The listing builds one solid part. Answer for the finished solid, in the listing's coordinates (mm). Coordinates: 2 decimals unless noted, no trailing zeros. Loops run counter-clockwise (first coordinate to the right, second up) from the corner with the lowest first, then second, coordinate; pieces in that order, holes last. Notation, with made-up numbers: (-2.75, -14.5) - (52.25, -14.5) arc R23 ccw to (52.25, 24.5) - close; hole circle Ø9 at (-29, 34.25). An arc over 180 degrees is marked (long way). Use one line per item in the form item = value. Start each with the question number.
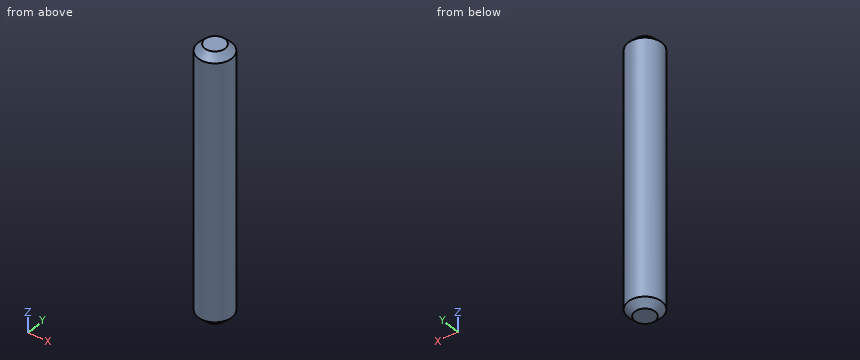
```python
from build123d import *

# Parameters (mm, degrees)
SKETCH_1_R      = 2.5
EXTRUDE_1_DEPTH = 40
CHAMFER_1_SIZE  = 1
CHAMFER_2_SIZE  = 1


with BuildPart() as part:
    # Эскиз1 → Бобышка-Вытянуть1 (new body)
    with BuildSketch(Plane.XY):
        Circle(SKETCH_1_R)
    extrude(amount=EXTRUDE_1_DEPTH)

    # Фаска1
    chamfer_1_edges = [part.edges().sort_by_distance(p)[0] for p in [
        (-2.5, 0, 40),
    ]]
    chamfer(chamfer_1_edges, length=CHAMFER_1_SIZE)

    # Фаска2
    chamfer_2_edges = [part.edges().sort_by_distance(p)[0] for p in [
        (-2.5, 0, 0),
    ]]
    chamfer(chamfer_2_edges, length=CHAMFER_2_SIZE)


solid = part.part
```
(1) Find the intervals of material crossed by probe 1 along X at (y, z) = (0.2, 27); probe 2 along Z at (x, y) = (-1.15, -2); probe 3 along Z at (x, y) = (-1.9, 0.8), in increasing order. Write a range as from..to.
(2) This flat-tipped pin is pushed along its axis until it touches: pin 1 Ø3 at (x, y) = (2, -1) entering from -Z. Where does it stop, or does it pass through?
(3) A cutting plane is placed at A-A (z = 3). Determine the outline of the cut face in (x, y), then the cut area to 3 significant figures.
Evaluation:
q1.probe_1 = -2.49..2.49
q1.probe_2 = 0.81..39.19
q1.probe_3 = 0.56..39.44
q2.pin_1 = 0
q3.outline = circle Ø5 at (0, 0)
q3.area = 19.6 mm^2
